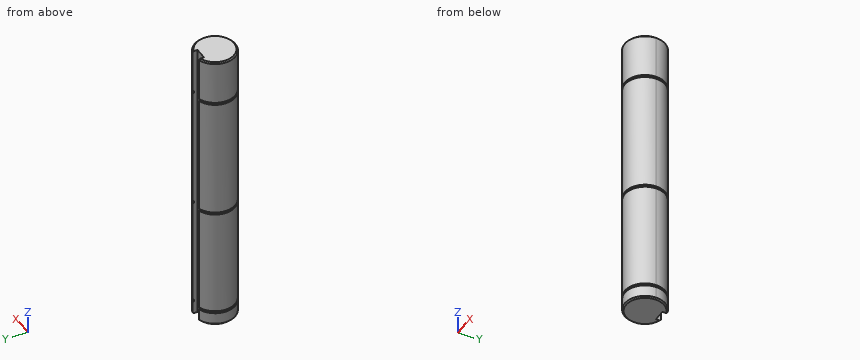
from build123d import *

# Parameters (mm, degrees)
BOSS_EXTRUDE1_DEPTH = 114.3
CHAMFER1_SIZE       = 0.508
SKETCH2_R           = 8.697781756
SKETCH2_R_2         = 7.366
CUT_EXTRUDE1_DEPTH  = 0.889
SKETCH3_OUTSIDE_W   = 41.162
SKETCH3_OUTSIDE_H   = 40.796
SKETCH3_OUTSIDE_R   = 7.366
CUT_EXTRUDE2_DEPTH  = 0.889
SKETCH4_OUTSIDE_W   = 41.162
SKETCH4_OUTSIDE_H   = 40.796
SKETCH4_OUTSIDE_R   = 7.366
CUT_EXTRUDE3_DEPTH  = 0.889


with BuildPart() as part:
    # Sketch1 → Boss-Extrude1 (new body)
    with BuildSketch(Plane.XY):
        with BuildLine():
            ThreePointArc((7.9375, 0), (6.399417088, 4.695888328), (2.38125, 7.571892411))
            Line((2.38125, 7.571892411), (2.38125, 5.55625))
            Line((2.38125, 5.55625), (-2.38125, 5.55625))
            Line((-2.38125, 5.55625), (-2.38125, 7.571892411))
            ThreePointArc((-2.38125, 7.571892411), (-4.695888328, -6.399417088), (7.9375, 0))
        make_face()
    extrude(amount=BOSS_EXTRUDE1_DEPTH)

    # Chamfer1
    chamfer1_edges = [part.edges().sort_by_distance(p)[0] for p in [
        (-4.695888328, -6.399417088, 0),
        (-4.695888328, -6.399417088, 114.3),
    ]]
    chamfer(chamfer1_edges, length=CHAMFER1_SIZE)

    # Sketch2 → Cut-Extrude1 (cut)
    with BuildSketch(Plane(origin=(0, 0, 5.08), x_dir=(-1, 0, 0), z_dir=(0, 0, -1))):
        Circle(SKETCH2_R)
        Circle(SKETCH2_R_2, mode=Mode.SUBTRACT)
    extrude(amount=-CUT_EXTRUDE1_DEPTH, mode=Mode.SUBTRACT)

    # Sketch3 outside → Cut-Extrude2 (cut)
    with BuildSketch(Plane.XY.offset(49.022)):
        with Locations((0, -0.183)):
            Rectangle(SKETCH3_OUTSIDE_W, SKETCH3_OUTSIDE_H)
        Circle(SKETCH3_OUTSIDE_R, mode=Mode.SUBTRACT)
    extrude(amount=-CUT_EXTRUDE2_DEPTH, mode=Mode.SUBTRACT)

    # Sketch4 outside → Cut-Extrude3 (cut)
    with BuildSketch(Plane.XY.offset(96.901)):
        with Locations((0, -0.183)):
            Rectangle(SKETCH4_OUTSIDE_W, SKETCH4_OUTSIDE_H)
        Circle(SKETCH4_OUTSIDE_R, mode=Mode.SUBTRACT)
    extrude(amount=-CUT_EXTRUDE3_DEPTH, mode=Mode.SUBTRACT)


solid = part.part
Geometry check sheet. Reference: the model listing, model coordinates, mm. Round coordinates to 2 decimals unless told otherwise and drop trailing zeros. Write each loop counter-clockwise with the first axis right and the second up, starting at its lowest first coordinate (ties: lowest second). Pieces come first, ordered by that corner, then holes.
Item 1: Material ranges on line 1 along Z through (x, y) = (5.75, -5.25); line 2 along X through (y, z) = (-2.75, 101.5); line 3 along X through (y, z) = (6, 97.5), recorded low to high.
Determined:
line 1: z = 0.36 to 5.08, 5.97 to 48.13, 49.02 to 96.01, 96.9 to 113.94
line 2: x = -7.45 to 7.45
line 3: x = -5.2 to -2.38, 2.38 to 5.2
Item 2: Section check A-A (x = 0). Record the boundary of the cut face in (y, z), plus the area to 3 significant figures.
Determined:
outline: (-7.94, 0.51) - (-7.43, 0) - (5.56, 0) - (5.56, 114.3) - (-7.43, 114.3) - (-7.94, 113.79) - (-7.94, 96.9) - (-7.37, 96.9) - (-7.37, 96.01) - (-7.94, 96.01) - (-7.94, 49.02) - (-7.37, 49.02) - (-7.37, 48.13) - (-7.94, 48.13) - (-7.94, 5.97) - (-7.37, 5.97) - (-7.37, 5.08) - (-7.94, 5.08) - close
area: 1,540 mm2
Item 3: Section check B-B (z = 18). Record the boundary of the cut face in (x, y) (1 decimal), plus the area to 3 significant figures.
Determined:
outline: (-2.4, 5.6) - (-2.4, 7.6) arc R7.9 ccw (long way) to (2.4, 7.6) - (2.4, 5.6) - close
area: 187 mm2
Item 4: Go/stop test with flat-tipped pins: pin 1 Ø3 at (y, z) = (5.5, 18.5) entering from -X; pin 2 Ø2 at (x, z) = (5.5, 73) entering from +Y; pin 3 Ø0.6 at (y, z) = (6.5, 76.5) entering from -X. Record where each tip stops, or that it passes through.
Determined:
pin 1: stops at x = -6.86
pin 2: stops at y = 6.54
pin 3: stops at x = -4.96
